Autodesk Inventor part; units mm, degrees
ref_plane "YZ Plane" through (0, 0, 0) normal (1, 0, 0) x (0, 1, 0)
ref_plane "XZ Plane" through (0, 0, 0) normal (0, 1, 0) x (-1, 0, 0)
ref_plane "XY Plane" through (0, 0, 0) normal (0, 0, 1) x (1, 0, 0)
sketch "Skizze3" plane through (0, 0, 0) normal (0, 0, 1) x (1, 0, 0)
  line L0 (-22.75, 0) -> (22.75, 0)
  line L1 (0, -17) -> (0, 11)
  line L2 (-16.25, 7) -> (0, 7)
  line L3 (16.25, 0) -> (16.25, -13)
  line L4 (16.25, -13) -> (-16.25, -13)
  line L5 (-16.25, -13) -> (-16.25, 7)
  line L6 (0, 7) -> (0, 0)
  line L7 (16.25, 0) -> (0, 0)
  point P0 (16.25, 0)
  point P1 (0, 7)
  dimension "d4" = 20
  dimension "d5" = 32.5
  dimension "d41" = 7
extrude "Extrusion3" add sketch "Skizze3" along normal blind 20
sketch "Skizze6" plane through (0, 0, 0) normal (0, 1, 0) x (1, 0, 0)
  line L0 (16.25, 0) -> (0, 0)
  line L1 (16.25, 0) -> (16.25, -20)
  circle A0 centre (8.25, -10) radius 1
  dimension "d21" = 10
  dimension "d22" = 8
  dimension "d23" = 2
extrude "Extrusion6" cut sketch "Skizze6" against normal blind 3
sketch "Skizze7" plane through (0, 0, 0) normal (1, 0, 0) x (0, 0, -1)
  line L0 (0, 0) -> (0, 7)
  line L1 (0, 7) -> (-20, 7)
  circle A0 centre (-10, 3.5) radius 1
  dimension "d26" = 10
  dimension "d27" = 3.5
  dimension "d28" = 2
extrude "Extrusion7" cut sketch "Skizze7" against normal blind 10
chamfer "Fase4" distance 2 angle 45 13 edges at (-8.125, 7, 20) (-16.25, -3, 20) (-16.25, 7, 10) (-16.25, -3, 0) (-8.125, 7, 0) (0, 7, 10) (8.125, 0, 0) (8.125, 0, 20) (16.25, 0, 10) (16.25, -6.5, 0) (16.25, -6.5, 20) (0, 3.5, 20) (0, 3.5, 0)
sketch "Skizze9" plane through (-14.25, -13, 0) normal (0, -1, 0) x (1, 0, 0)
  circle A0 centre (22.5, 10) radius 1
  line L0 (-2, 2) -> (-2, 18)
  point P0 (14.25, 0)
hole "Bohrung1" at (8.25, -13, 10) direction (0, 1, 0) diameter 11.445 depth 12
sketch "Skizze10" plane through (-14.25, -13, 0) normal (0, -1, 0) x (1, 0, 0)
  line L0 (0, 0) -> (28.5, 0)
  line L1 (-2, 2) -> (-2, 18)
  point P0 (14.25, 0)
  point P1 (6, 10)
  dimension "d53" = 10
  dimension "d54" = 8
hole "Bohrung2" at (-8.25, -13, 10) direction (0, 1, 0) diameter 11.445 depth 18
properties part number "1"
Could you check a few things on this model? Use its own coordinates, in mm. A direction names the side the tool comes from. Round coordinates to 2 decimals unless told otherwise and drop trailing zeros. Order: outer loops, then holes, each group sorted by start corner. A loop starts at its lowest first (then second) coordinate and runs counter-clockwise, first axis right, second up. Notation, with made-up numbers: M 81,22 L 114,22 A17 ccw 114,52 Z; hole C 45.25,38 d7. An arc over 180 degrees is marked long. One line per item, written item: value.
(1) If we mould it in two halves opening along Z, with no side actions, what happens to faces 1 (the flat face through (-16.25, -4, 10)), 2 (the cylindrical face through (8.12, -0.49, 9.01)), 3 (the flat face through (15.014, -1.368, 1.396))? For each: released by +Z, released by -Z, zero draft, split by the parting line, or undercut.
Ans:
face 1: zero draft
face 2: undercut
face 3: released by -Z
(2) Imagine slicing it at D-D (y = -3). Count the separate pieces of the cut face and the enclosed holes in it, and give its area (3 significant figures).
Ans:
separate pieces: 1
enclosed holes: 2
area: 436 mm^2
(3) Imagine slicing it at B-B (x = 8.25). Write out the boundary of the cut face in (y, z), and give its area (3 significant figures).
Ans:
outline: M -13,0 L -2,0 L 0,2 L 0,9 L -1,9 L -1,4.28 L -13,4.28 Z; M -13,15.72 L -1,15.72 L -1,11 L 0,11 L 0,18 L -2,20 L -13,20 Z
area: 117 mm^2
(4) Which directions (+Z, -Z, +X, -X, +Y, -Y) give clear straight access to the entire face, cutting with the end or side of a thin tool? Please do faces 4 (the flat face through (7, 0, 10)), 5 (the flat face through (-8, 5, 10)), 6 (the flat face through (6, -1, 19)), 7 (the flat face through (-15.24, 6.01, 9.89)), 8 (the flat face through (-1, 2, 1)).
Ans:
face 4: +Z, -Z, +X, +Y
face 5: -Y
face 6: +Z, +X, +Y
face 7: +Z, -Z, -X, +Y
face 8: -Z, +X, +Y
(5) Imagine slicing it at A-A (z = 10). Write out the boundary of the cut face in (x, y).
Ans:
outline: M -16.25,-13 L -13.97,-13 L -13.97,5 L -2.53,5 L -2.53,4.5 L 0,4.5 L 0,5 L -2,7 L -14.25,7 L -16.25,5 Z; M -2.53,-13 L 2.53,-13 L 2.53,-1 L 7.25,-1 L 7.25,0 L 0,0 L 0,2.5 L -2.53,2.5 Z; M 9.25,-1 L 13.97,-1 L 13.97,-13 L 16.25,-13 L 16.25,-2 L 14.25,0 L 9.25,0 Z
(6) I need wall thicknesses on line 1 along X through (y, z) = (-8, 10); line 2 along Z through (x, y) = (-8.25, -4); line 3 along X through (y, z) = (-2.25, 6.5). Which ranges of each line are inside material? Lowest first, please. Write a range as from..to.
Ans:
line 1: x = -16.25..-13.97, -2.53..2.53, 13.97..16.25
line 2: z = 0..4.28, 15.72..20
line 3: x = -16.25..-12.78, -3.72..3.72, 12.78..16.25
(7) I'm going to push flat-ended pins straight in: P1, Ø2.5, axis at x = 8.25, z = 10, coming from the -Y side; P2, Ø3.5, axis at x = -6.5, z = 10.5, coming from the -Y side; P3, Ø8, axis at x = 5, z = 3, coming from the +Y side. Where does each tip first touch, or does it pass through?
Ans:
P1: stops at y = -1
P2: stops at y = 5
P3: stops at y = 0
